from build123d import *

# Parameters (mm, degrees)
F0_R     = 6.75
F1_DEPTH = 8
F3_DEPTH = 8.001


with BuildPart() as f1:
    # F0 (on Top) → F1 (new body)
    with BuildSketch(Plane.XY):
        Circle(F0_R)
    extrude(amount=F1_DEPTH)

    # F2 (on face) → F3 (cut, through all)
    with BuildSketch(Plane(origin=(0, 0, 0), x_dir=(1, 0, 0), z_dir=(0, 0, -1))):
        with BuildLine():
            Line((1.106261084, 1.0130085952), (4.0290932015, 3.7438493524))
            ThreePointArc((4.0290932015, 3.7438493524), (2.1975928378, 5.0418831521), (0, 5.5))
            Line((0, 5.5), (0, 1.5))
            ThreePointArc((0, 1.5), (0.6043538315, 1.3728643219), (1.106261084, 1.0130085952))
        make_face()
        with BuildLine():
            Line((-1.0654173052, 1.055881606), (-3.8317758444, 3.9455663571))
            ThreePointArc((-3.8317758444, 3.9455663571), (-5.0658053231, 2.1418721783), (-5.5, 0))
            Line((-5.5, 0), (-1.5, 0))
            ThreePointArc((-1.5, 0), (-1.3871059725, 0.5709089429), (-1.0654173052, 1.055881606))
        make_face()
        with BuildLine():
            ThreePointArc((-4.0085548388, -3.7658316617), (-2.1837955331, -5.0478745101), (0, -5.5))
            Line((0, -5.5), (0, -1.5))
            ThreePointArc((0, -1.5), (-0.5905563661, -1.3788557497), (-1.0857227213, -1.0349909046))
            Line((-1.0857227213, -1.0349909046), (-4.0085548388, -3.7658316617))
        make_face()
        with BuildLine():
            ThreePointArc((3.7747972956, -4.0001131705), (5.0503160855, -2.1781431167), (5.5, 0))
            Line((5.5, 0), (1.5, 0))
            ThreePointArc((1.5, 0), (1.3716154954, -0.6071827836), (1.0084387564, -1.1104284194))
            Line((1.0084387564, -1.1104284194), (3.7747972956, -4.0001131705))
        make_face()
    extrude(amount=-F3_DEPTH, mode=Mode.SUBTRACT)


solid = f1.part
Check sheet for the modelled part. Datum: model origin and axes. Units: mm. A direction names the side the tool comes from. Round coordinates to 2 decimals unless told otherwise and drop trailing zeros. Order: outer loops, then holes, each group sorted by start corner. A loop starts at its lowest first (then second) coordinate and runs counter-clockwise, first axis right, second up.
(1) Cross-section at D-D, the plane y = 3. Enter the section's corners in (x, z).
(2) Access from +Z, -Z, +X, -X, +Y, -Y to the whole of each face (thin tool, end or side, straight path). Record for faces 1 (the cylindrical face through (-1.39, -0.56, 3.94)), 2 (the flat face through (0, 0, 0)).
(3) Go/stop test with flat-tipped pins: P1, Ø3, axis at x = 5, z = 4.5, coming from the +Y side; P2, Ø1, axis at x = -3, z = 4, coming from the -Y side; P3, Ø3, axis at x = -4.5, z = 5.5, coming from the -Y side; P4, Ø1.5, axis at x = -2.5, y = 0, coming from the -Z side. Record where each tip stops, or that it passes through.
(4) Cross-section at B-B, the plane x = 0.25. Enter the section's corners in (y, z).
(5) Cross-section at C-C, the plane x = 3.5. Enter the section's corners in (y, z).
(6) Cross-section at A-A, the plane z = 0.5. Enter the section's corners in (x, y) (3 decimals).
(7) Scan lines: probe 1 along Y at (x, z) = (-1.25, 6); probe 2 along Y at (x, z) = (2, 5.75); probe 3 along X at (y, z) = (-3.5, 2.5). Record each from-to range of solid material in increasing order.
(8) Draft check along Y on faces 3 (the cylindrical face through (-1.46, -6.59, 3.94)), 4 (the cylindrical face through (-0.583, 1.382, 3.944)), 5 (the flat face through (0, 0, 8)). Enter one of: pulls with the +Y half, pulls with the -Y half, needs draft (parallel to the pull), parting line crosses it, or undercut.
Check sheet entries:
1. outline: (-6.05, 0) - (-3.19, 0) - (-3.19, 8) - (-6.05, 8) - close; (0, 0) - (2.82, 0) - (2.82, 8) - (0, 8) - close; (4.61, 0) - (6.05, 0) - (6.05, 8) - (4.61, 8) - close
2. face 1: +Z, -Z
2. face 2: -Z, +X, -X, +Y, -Y
3. P1: stops at y = 5.77
3. P2: stops at y = -6.27
3. P3: stops at y = -6.05
3. P4: stops at z = 0
4. outline: (-6.75, 0) - (-5.49, 0) - (-5.49, 8) - (-6.75, 8) - close; (-1.48, 0) - (6.75, 0) - (6.75, 8) - (-1.48, 8) - close
5. outline: (-5.77, 0) - (-4.24, 0) - (-4.24, 8) - (-5.77, 8) - close; (-3.25, 0) - (0, 0) - (0, 8) - (-3.25, 8) - close; (3.71, 0) - (5.77, 0) - (5.77, 8) - (3.71, 8) - close
6. outline: circle Ø13.5 at (0, 0); hole (-5.5, 0) arc R5.5 ccw to (-3.832, -3.946) - (-1.065, -1.056) arc R1.5 cw to (-1.5, 0) - close; hole (-4.009, 3.766) - (-1.086, 1.035) arc R1.5 cw to (0, 1.5) - (0, 5.5) arc R5.5 ccw to start; hole (0, -5.5) arc R5.5 ccw to (4.029, -3.744) - (1.106, -1.013) arc R1.5 cw to (0, -1.5) - close; hole (1.008, 1.11) arc R1.5 cw to (1.5, 0) - (5.5, 0) arc R5.5 ccw to (3.775, 4) - close
7. probe 1: y = -6.63 to -1.25, -0.83 to 1.19, 5.36 to 6.63
7. probe 2: y = -6.45 to -5.12, -1.85 to 0, 2.15 to 6.45
7. probe 3: x = -5.77 to -4.24, -3.41 to 0, 3.77 to 5.77
8. face 3: parting line crosses it
8. face 4: undercut
8. face 5: needs draft
